from build123d import *

# Parameters (mm, degrees)
SKETCH1_R           = 2.286
SKETCH1_R_2         = 2.667
BOSS_EXTRUDE1_DEPTH = 10.16
SKETCH7_R           = 3.6195
SKETCH7_R_2         = 4.6355
CUT_EXTRUDE1_DEPTH  = 4.064
SKETCH3_R           = 1.397
CUT_EXTRUDE2_DEPTH  = 1.016
SKETCH8_R           = 1.397
CUT_EXTRUDE3_DEPTH  = 1.016
CUT_EXTRUDE4_START  = -1.016
SKETCH9_R           = 1.397
CUT_EXTRUDE4_DEPTH  = 1.016
FILLET1_R           = 1.27


with BuildPart() as part:
    # Sketch1 → Boss-Extrude1 (new body)
    with BuildSketch(Plane.XY):
        Polygon((0, 57.15), (10.16, 57.15), (10.16, 67.31), (22.86, 67.31), (22.86, 57.15), (33.02, 57.15), (33.02, 0), (0, 0), align=None)
        with Locations((5.08, 7.62)):
            Circle(SKETCH1_R, mode=Mode.SUBTRACT)
        with Locations((5.08, 30.48)):
            Circle(SKETCH1_R, mode=Mode.SUBTRACT)
        with Locations((26.67, 15.24)):
            Circle(SKETCH1_R_2, mode=Mode.SUBTRACT)
        with Locations((22.86, 30.48)):
            Circle(SKETCH1_R, mode=Mode.SUBTRACT)
    extrude(amount=BOSS_EXTRUDE1_DEPTH)

    # Sketch7 → Cut-Extrude1 (cut)
    with BuildSketch(Plane.XY.offset(10.16)):
        with Locations((5.08, 30.48)):
            Circle(SKETCH7_R)
        with Locations((22.86, 30.48)):
            Circle(SKETCH7_R)
        with Locations((5.08, 7.62)):
            Circle(SKETCH7_R)
        with Locations((26.67, 15.24)):
            Circle(SKETCH7_R_2)
    extrude(amount=-CUT_EXTRUDE1_DEPTH, mode=Mode.SUBTRACT)

    # Sketch3 → Cut-Extrude2 (cut)
    with BuildSketch(Plane(origin=(0, 0, 10.16), x_dir=(-1, 0, 0), z_dir=(0, 0, -1))):
        with Locations((-16.51, 62.23)):
            Circle(SKETCH3_R)
    extrude(amount=CUT_EXTRUDE2_DEPTH, mode=Mode.SUBTRACT)

    # Sketch8 → Cut-Extrude3 (cut)
    with BuildSketch(Plane(origin=(22.86, 0, 0), x_dir=(0, 0, -1), z_dir=(1, 0, 0))):
        with Locations((-5.08, 62.23)):
            Circle(SKETCH8_R)
    extrude(amount=-CUT_EXTRUDE3_DEPTH, mode=Mode.SUBTRACT)

    # Sketch9 → Cut-Extrude4 (cut)
    with BuildSketch(Plane.ZY.offset(-10.16).offset(CUT_EXTRUDE4_START)):
        with Locations(Location((5.08, 62.23, 0), (0, 0, 180))):
            Circle(SKETCH9_R)
    extrude(amount=CUT_EXTRUDE4_DEPTH, mode=Mode.SUBTRACT)

    # Fillet1
    fillet1_edges = [part.edges().sort_by_distance(p)[0] for p in [
        (33.02, 28.575, 10.16),
        (0, 57.15, 5.08),
        (33.02, 57.15, 5.08),
        (33.02, 0, 5.08),
        (0, 0, 5.08),
        (0, 28.575, 10.16),
        (16.51, 0, 10.16),
        (33.02, 28.575, 0),
    ]]
    fillet(fillet1_edges, radius=FILLET1_R)


solid = part.part
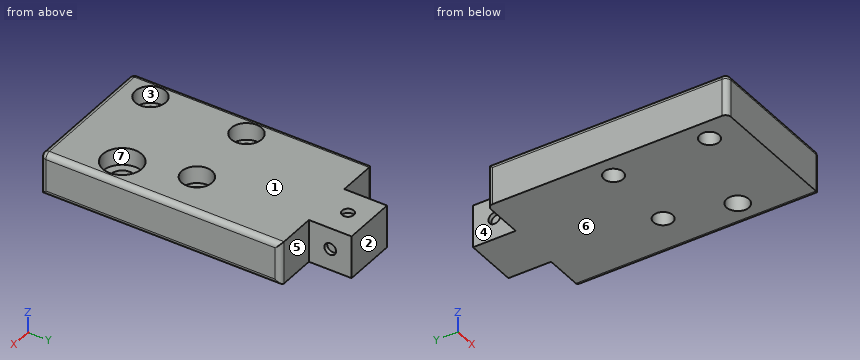
The listing builds one solid part. Answer for the finished solid, in the listing's coordinates (mm). Face numbers are marked on the shaded views. A direction names the side the tool comes from. Give positions to 0.01 mm unless a question says otherwise; leave off trailing zeros. Loops run counter-clockwise (first coordinate to the right, second up) from the corner with the lowest first, then second, coordinate; pieces in that order, holes last. Notation, with made-up numbers: (-20, 85.25) - (-13, 85.25) arc R13 ccw to (-13, 92.25) - close; hole circle Ø2 at (-31.5, 42.25). An arc over 180 degrees is marked (long way). Answer as a JSON object with one key per item and string values.
1. For a pull along Y with two mould halves and no side action, classify the marked faces 1, 2 and 3 as pulls with the +Y half, pulls with the -Y half, needs draft (parallel to the pull), parting line crosses it, or undercut.
Determined:
{"face 1": "needs draft", "face 2": "pulls with the +Y half", "face 3": "undercut"}
2. A cutting plane is placed at D-D (x = 6.5). Write down the section's boundary in (y, z).
Determined:
{"outline": "(0, 0) - (5.83, 0) - (5.83, 6.1) - (4.29, 6.1) - (4.29, 10.16) - (1.27, 10.16) arc R1.27 ccw to (0, 8.89) - close; (9.41, 0) - (28.69, 0) - (28.69, 6.1) - (27.15, 6.1) - (27.15, 10.16) - (10.95, 10.16) - (10.95, 6.1) - (9.41, 6.1) - close; (32.27, 0) - (57.15, 0) - (57.15, 10.16) - (33.81, 10.16) - (33.81, 6.1) - (32.27, 6.1) - close"}
3. A cutting plane is placed at C-C (y = 30.48). Write down the section's boundary in (x, z), then the cut area to 3 significant figures.
Determined:
{"outline": "(0, 0) - (2.79, 0) - (2.79, 6.1) - (1.46, 6.1) - (1.46, 10.16) - (1.27, 10.16) arc R1.27 ccw to (0, 8.89) - close; (7.37, 0) - (20.57, 0) - (20.57, 6.1) - (19.24, 6.1) - (19.24, 10.16) - (8.7, 10.16) - (8.7, 6.1) - (7.37, 6.1) - close; (25.15, 0) - (31.75, 0) arc R1.27 ccw to (33.02, 1.27) - (33.02, 8.89) arc R1.27 ccw to (31.75, 10.16) - (26.48, 10.16) - (26.48, 6.1) - (25.15, 6.1) - close", "area": "220 mm²"}
4. For the marked faces 4, 5, 6 and 7, determine the directions among +Z, -Z, +X, -X, +Y, -Y from which every point of the face is accessible in a straight line to the end or side of a thin tool.
Determined:
{"face 4": "+Z, -Z, -X, +Y", "face 5": "+Z, -Z, +X, +Y", "face 6": "-Z, +X, -X, +Y, -Y", "face 7": "+Z"}
5. A cutting plane is placed at A-A (y = 7.62). Write down the section's boundary in (x, z), then the cut area to 3 significant figures.
Determined:
{"outline": "(0, 0) - (2.79, 0) - (2.79, 6.1) - (1.46, 6.1) - (1.46, 10.16) - (1.27, 10.16) arc R1.27 ccw to (0, 8.89) - close; (7.37, 0) - (31.75, 0) arc R1.27 ccw to (33.02, 1.27) - (33.02, 8.89) arc R1.27 ccw to (31.75, 10.16) - (8.7, 10.16) - (8.7, 6.1) - (7.37, 6.1) - close", "area": "277 mm²"}
6. Flat-ended cylindrical pins translate along their axes: pin 1 Ø1 at (y, z) = (60, 6) entering from +X; pin 2 Ø4.5 at (y, z) = (62.23, 5.08) entering from -X; pin 3 Ø6 at (x, y) = (5.08, 30.48) entering from +Z; pin 4 Ø3 at (x, y) = (26.67, 15.24) entering from +Z. Find the tip coordinate at first contact, or state that the pin passes through.
Determined:
{"pin 1": "x = 22.86", "pin 2": "x = 10.16", "pin 3": "z = 6.1", "pin 4": "through"}
7. A cutting plane is placed at B-B (z = 5.08). Write down the section's boundary in (x, y).
Determined:
{"outline": "(0, 1.27) arc R1.27 ccw to (1.27, 0) - (31.75, 0) arc R1.27 ccw to (33.02, 1.27) - (33.02, 55.88) arc R1.27 ccw to (31.75, 57.15) - (22.86, 57.15) - (22.86, 60.83) - (21.84, 60.83) - (21.84, 63.63) - (22.86, 63.63) - (22.86, 67.31) - (10.16, 67.31) - (10.16, 63.63) - (11.18, 63.63) - (11.18, 60.83) - (10.16, 60.83) - (10.16, 57.15) - (1.27, 57.15) arc R1.27 ccw to (0, 55.88) - close; hole circle Ø4.57 at (5.08, 7.62); hole circle Ø4.57 at (5.08, 30.48); hole circle Ø4.57 at (22.86, 30.48); hole circle Ø5.33 at (26.67, 15.24)"}
8. Find the intervals of material crossed by L1, parallel to Y at x = 5.08, z = 7.35; L2, parallel to Y at x = 10.6, z = 5.08; L3, parallel to Y at x = 23, z = 2.5, in increasing order. Write a range as [from, to].
Determined:
{"L1": "[0, 4], [11.24, 26.86], [34.1, 57.15]", "L2": "[0, 60.83], [63.63, 67.31]", "L3": "[0, 28.2], [32.76, 57.15]"}
